Design review of the part shown in the three views and the two pictorial views. Dimensions are in mm from the part's minimum x, y and z. A direction names the side the tool comes from. Round coordinates to 2 decimals unless told otherwise and drop trailing zeros. Order: outer loops, then holes, each group sorted by start corner. A loop starts at its lowest first (then second) coordinate and runs counter-clockwise, first axis right, second up. Notation, with made-up numbers: M 57.5,69 L 75.5,69 A25 ccw 75.5,106 Z; hole C 3.25,-39.75 d4. An arc over 180 degrees is marked long. Write each question's results on one line, items separated by ' | '. Start each with the question number.
Item 1: The part is to be moulded in two halves that separate along Y. For the marked faces 5 and 6, say which applies: +Y half, -Y half, draft (parallel to the pull), parting line (faces both ways), or undercut.
Item 2: Wall thickness on line 1 (Y direction, x = 56, z = 0.95) (3 decimals); line 2 (X direction, y = 7.5, z = 1.3) (3 decimals); line 3 (X direction, y = 30, z = 1.65) (3 decimals): over which ranges is each line inside the solid? List them lowest first. Write a range as [from, to].
Item 3: Clearance check with flat-ended pins moving along their axes: pin 1 (1.2 mm diameter, centred on x = 18, z = 1.5, fed in from +Y); pin 2 (3.5 mm diameter, centred on x = 12, y = 31.5, fed in from -Z); pin 3 (2 mm diameter, centred on y = 42.5, z = 1, fed in from +X). State where each tip first meets the part, or that it passes through.
Item 4: Take a section at C-C, the plane y = 40. Write out the cut boundary in (x, z) (3 decimals), plus the area to 3 significant figures.
Item 5: Take a section at D-D, the plane x = 54.5. Write out the cut boundary in (y, z) (3 decimals).
Item 6: Take a section at B-B, the plane z = 1.3. Write out the cut boundary in (x, y) (3 decimals).
Item 7: Take a section at A-A, the plane x = 48. Write out the cut boundary in (y, z) (3 decimals).
Item 8: Machinability: for the marked faces 1, 2, 3 and 4, which of the approach directions +Z, -Z, +X, -X, +Y, -Y give a long, thin tool a straight path to every point of the face, cutting with its end or side? Answer none if there is none.
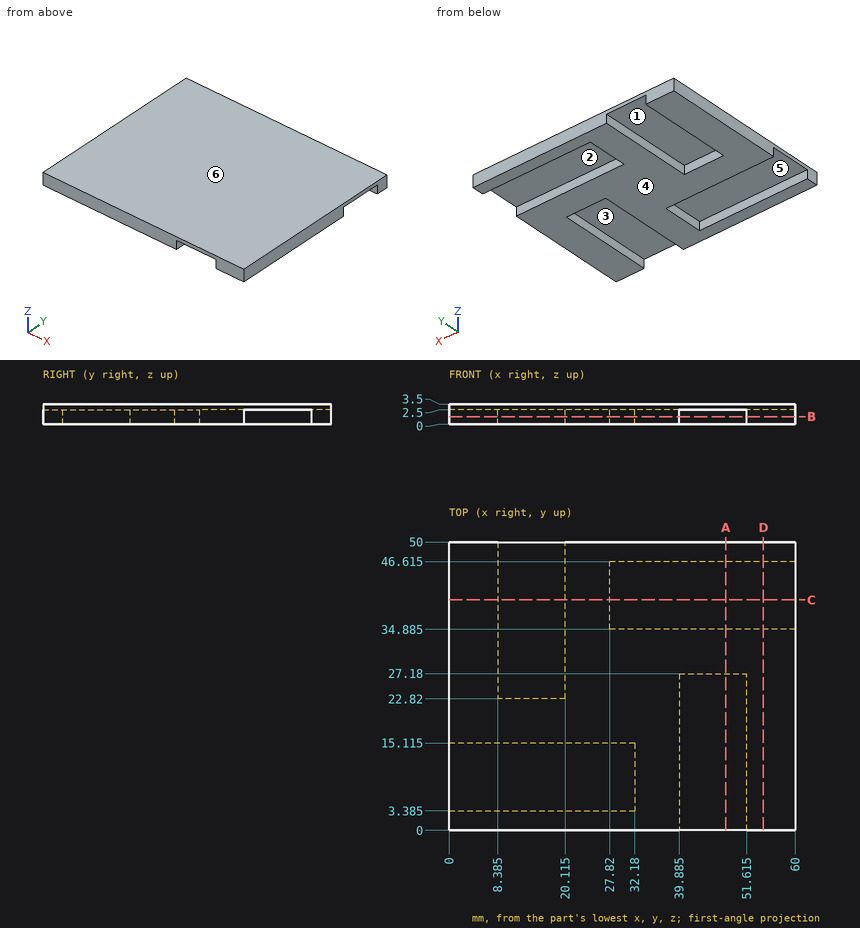
Results list:
1) face 5: undercut | face 6: draft
2) line 1: [0, 34.885], [46.615, 50] | line 2: [32.18, 39.885], [51.615, 60] | line 3: [0, 8.385], [20.115, 60]
3) pin 1: y = 22.82 | pin 2: z = 2.5 | pin 3: x = 27.82
4) outline: M 0,0 L 8.385,0 L 8.385,2.5 L 20.115,2.5 L 20.115,0 L 27.82,0 L 27.82,2.5 L 60,2.5 L 60,3.5 L 0,3.5 Z | area: 100 mm²
5) outline: M 0,0 L 34.885,0 L 34.885,2.5 L 46.615,2.5 L 46.615,0 L 50,0 L 50,3.5 L 0,3.5 Z
6) outline: M 0,0 L 39.885,0 L 39.885,27.18 L 51.615,27.18 L 51.615,0 L 60,0 L 60,34.885 L 27.82,34.885 L 27.82,46.615 L 60,46.615 L 60,50 L 20.115,50 L 20.115,22.82 L 8.385,22.82 L 8.385,50 L 0,50 L 0,15.115 L 32.18,15.115 L 32.18,3.385 L 0,3.385 Z
7) outline: M 0,2.5 L 27.18,2.5 L 27.18,0 L 34.885,0 L 34.885,2.5 L 46.615,2.5 L 46.615,0 L 50,0 L 50,3.5 L 0,3.5 Z
8) face 1: -Z, +Y | face 2: -Z, +X | face 3: -Z, -Y | face 4: -Z, +X, -X, +Y, -Y
